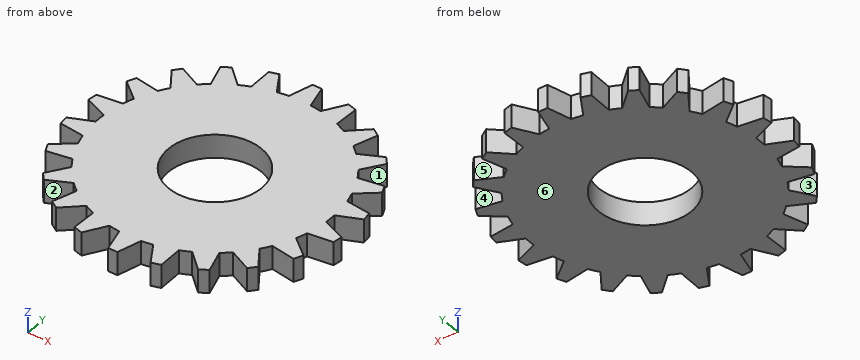
```python
from build123d import *

# Parameters (mm, degrees)
F0_R            = 12.7
F0_R_2          = 5.08
F1_DEPTH        = 2.54
F3_DEPTH        = 2.54
F3_COPIES_COUNT = 22


# Not quite as in the source:
# - a pattern or mirror of a feature is missing from the dataset's text; its kind, count and spacing are read off the source's solid
# - a feature names something its author has since deleted; it is built from what else it names


with BuildPart() as f1:
    # F0 (on Top) → F1 (new body)
    with BuildSketch(Plane.XY):
        Circle(F0_R)
        Circle(F0_R_2, mode=Mode.SUBTRACT)
    extrude(amount=F1_DEPTH)

    # F2 (on face) → F3 (join)
    with BuildSketch(Plane.XY.offset(2.54)):
        with BuildLine():
            ThreePointArc((-1.2039155713, 12.64280773), (0, 12.7), (1.2039155713, 12.64280773))
            Line((1.2039155713, 12.64280773), (0.508, 15.24))
            Line((0.508, 15.24), (0, 15.24))
            Line((0, 15.24), (-0.508, 15.24))
            Line((-0.508, 15.24), (-1.2039155713, 12.64280773))
        make_face()
    f3 = extrude(amount=-F3_DEPTH)

    # F3_copies: F3 ×22 about axis
    f3_copies_axis = Axis((0, 0, 0), (0, 0, 1))
    for i in range(1, F3_COPIES_COUNT):
        add(f3.rotate(f3_copies_axis, i * 360 / F3_COPIES_COUNT))


solid = f1.part
```
Can you work these out from the model? Positions are in its coordinate system, mm. Face numbers are marked on the shaded views. A direction names the side the tool comes from. Round coordinates to 2 decimals unless told otherwise and drop trailing zeros. Order: outer loops, then holes, each group sorted by start corner. A loop starts at its lowest first (then second) coordinate and runs counter-clockwise, first axis right, second up. Notation, with made-up numbers: (-36.75, 62.5) -> (-25.75, 62.5) arc R13 cw to (-25.75, 82.5) -> close; hole circle Ø10 at (71.5, 0.25). An arc over 180 degrees is marked (long way). Return JSON: item names as keys, results as strings. Group by question number.
1. If we section it at A-A, the plane y = 0: Write out the boundary of the cut face in (x, z).
2. I need wall thicknesses on line 1 (Y direction, x = 0, z = 1.15); line 2 (Y direction, x = 14, z = 2.4); line 3 (Y direction, x = 13, z = 1.75). Which ranges of each line are inside material? Lowest first, please. Write a range as [from, to].
3. We'd pull the mould along Y, two halves only. Please class the marked faces 4, 5 and 6: released by +Y, released by -Y, zero draft, split by the parting line, or undercut.
4. Which directions (+Z, -Z, +X, -X, +Y, -Y) give clear straight access to the entire face, cutting with the end or side of a thin tool? Please do the marked faces 1, 2 and 3.
5. If we section it at C-C, the plane y = 5.5: Write out the boundary of the cut face in (x, z), then the cut area to 3 significant figures.
6. If we section it at B-B, the plane x = 0: Write out the boundary of the cut face in (y, z).
Output values:
{
 "1": {"outline": "(-12.7, 0) -> (-5.08, 0) -> (-5.08, 2.54) -> (-12.7, 2.54) -> close; (5.08, 0) -> (12.7, 0) -> (12.7, 2.54) -> (5.08, 2.54) -> close"},
 "2": {"line 1": "[-15.24, -5.08], [5.08, 15.24]", "line 2": "[-6.03, -5.81], [-2.79, -1.17], [1.17, 2.79], [5.81, 6.03]", "line 3": "[-6.68, -4.98], [-2.91, -0.74], [0.74, 2.91], [4.98, 6.68]"},
 "3": {"face 4": "undercut", "face 5": "released by +Y", "face 6": "zero draft"},
 "4": {"face 1": "+Z, -Z, +X", "face 2": "+Z, -Z, -Y", "face 3": "+Z, -Z, -X"},
 "5": {"outline": "(-13.63, 0) -> (13.63, 0) -> (13.63, 2.54) -> (-13.63, 2.54) -> close", "area": "69.2 mm²"},
 "6": {"outline": "(-15.24, 0) -> (-5.08, 0) -> (-5.08, 2.54) -> (-15.24, 2.54) -> close; (5.08, 0) -> (15.24, 0) -> (15.24, 2.54) -> (5.08, 2.54) -> close"}
}
